from build123d import *

# Parameters (mm, degrees)
ESQUISSE1_R             = 4.25
ESQUISSE1_R_2           = 2.5
BOSS_EXTRU_1_DEPTH      = 3
ESQUISSE1_4_R           = 2.5
BOSS_EXTRU_3_DEPTH      = 25
ENL_V_MAT_EXTRU_1_DEPTH = 1


with BuildPart() as part:
    # Esquisse1 → Boss.-Extru.1 (new body)
    with BuildSketch(Plane(origin=(0, 0, 0), x_dir=(1, 0, 0), z_dir=(0, 1, 0))):
        with Locations(Location((0, 0, 0), (0, 0, 270))):
            Circle(ESQUISSE1_R)
        with Locations(Location((0, 0, 0), (0, 0, 270))):
            Circle(ESQUISSE1_R_2, mode=Mode.SUBTRACT)
    extrude(amount=BOSS_EXTRU_1_DEPTH)

    # Esquisse1_4 → Boss.-Extru.3 (add)
    with BuildSketch(Plane(origin=(0, 0, 0), x_dir=(1, 0, 0), z_dir=(0, 1, 0))):
        with Locations(Location((0, 0, 0), (0, 0, 270))):
            Circle(ESQUISSE1_4_R)
    extrude(amount=BOSS_EXTRU_3_DEPTH)

    # Esquisse2 → Enl_v. mat.-Extru.1 (cut)
    with BuildSketch(Plane.XZ):
        Polygon((-1, 0), (-1, 8), (1, 8), (1, -8), (-1, -8), align=None)
    extrude(amount=-ENL_V_MAT_EXTRU_1_DEPTH, mode=Mode.SUBTRACT)


solid = part.part
Read the model definition and answer for the solid it produces. Units are mm, in the model's axes. A direction names the side the tool comes from. Give positions to 0.01 mm unless a question says otherwise; leave off trailing zeros. Write each loop counter-clockwise with the first axis right and the second up, starting at its lowest first coordinate (ties: lowest second). Pieces come first, ordered by that corner, then holes. Notation, with made-up numbers: (3.25, 24) - (56.25, 24) arc R7 ccw to (56.25, 35) - close; hole circle Ø7 at (-9.5, 23.5). An arc over 180 degrees is marked (long way). Use CSV: the item, a comma, the result in double quotes. Start each with the question number.
Item 1: The mould has two halves that part along X. Classify faces 4 (the flat face through (0, 25, 0)), 5 (the flat face through (0, 1, 0)), 6 (the cylindrical face through (-2.44, 13.85, -0.54)): pulls with the +X half, pulls with the -X half, needs draft (parallel to the pull), parting line crosses it, or undercut.
Item 2: For faces 1 (the flat face through (-1, 0.5, 0.1)), 2 (the flat face through (-2, 3, 2)), 3 (the cylindrical face through (1.277, 1.479, 4.054)), determine the directions among +Z, -Z, +X, -X, +Y, -Y from which every point of the face is accessible in a straight line to the end or side of a thin tool.
Item 3: The part is cut by section C-C, the plane y = 19. Give the vertices of the cut face in (x, z), and give its area (3 significant figures).
Item 4: The part is cut by section B-B, the plane x = 0. Give the vertices of the cut face in (y, z).
Item 5: The part is cut by section A-A, the plane z = 0. Give the vertices of the cut face in (x, y), and give its area (4 significant figures).
Item 6: Consider line 1 (Y direction, x = -2.25, z = -2.5); line 2 (Y direction, x = -0.75, z = 0); line 3 (Z direction, x = -1.5, y = 7.25). Determine where each line is inside the solid, lowest interval first.
Item 7: The part is cut by section D-D, the plane z = -2. Give the vertices of the cut face in (x, y), and give its area (3 significant figures).
Item 8: Flat-ended cylindrical pins translate along their axes: P1, Ø0.5, axis at y = 0.5, z = -1.5, coming from the +X side; P2, Ø3, axis at x = 3.5, z = -3, coming from the +Y side; P3, Ø0.6, axis at x = 0, z = 0, coming from the -Y side. Find the tip coordinate at first contact, or state that the pin passes through.
Taken from the geometry:
1,face 4,"needs draft"
1,face 5,"undercut"
1,face 6,"parting line crosses it"
2,face 1,"+Z, -Z, -Y"
2,face 2,"+Y"
2,face 3,"+Y, -Y"
3,outline,"circle Ø5 at (0, 0)"
3,area,"19.6 mm2"
4,outline,"(1, -4.25) - (3, -4.25) - (3, -2.5) - (25, -2.5) - (25, 2.5) - (3, 2.5) - (3, 4.25) - (1, 4.25) - close"
5,outline,"(-4.25, 0) - (-1, 0) - (-1, 1) - (1, 1) - (1, 0) - (4.25, 0) - (4.25, 3) - (2.5, 3) - (2.5, 25) - (-2.5, 25) - (-2.5, 3) - (-4.25, 3) - close"
5,area,"133.5 mm2"
6,line 1,"0 to 3"
6,line 2,"1 to 25"
6,line 3,"-2 to 2"
7,outline,"(-3.75, 0) - (-1, 0) - (-1, 1) - (1, 1) - (1, 0) - (3.75, 0) - (3.75, 3) - (1.5, 3) - (1.5, 25) - (-1.5, 25) - (-1.5, 3) - (-3.75, 3) - close"
7,area,"86.5 mm2"
8,P1,"x = 4.06"
8,P2,"y = 3"
8,P3,"y = 1"
